Verification items for the finished model (mm, model axes). Face numbers are marked on the shaded views. A direction names the side the tool comes from. Coordinates: 2 decimals unless noted, no trailing zeros. Write each loop counter-clockwise with the first axis right and the second up, starting at its lowest first coordinate (ties: lowest second). Pieces come first, ordered by that corner, then holes. Notation, with made-up numbers: M 57,-36.5 L 91,-36.5 A7 ccw 91,-28.5 Z; hole C 14,-34 d1. An arc over 180 degrees is marked long. One line per item, written item: value.
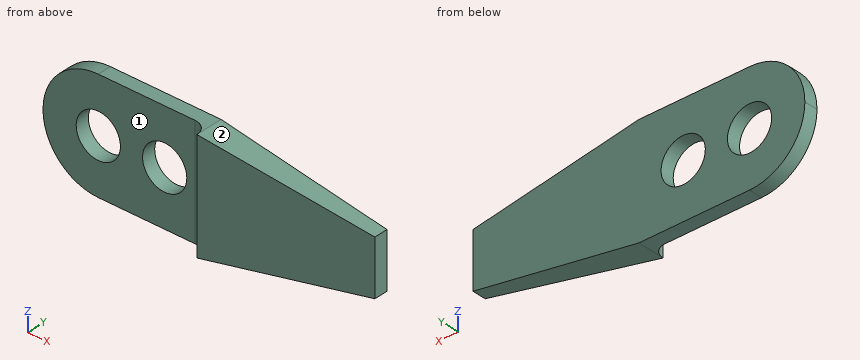
```python
from build123d import *

# Parameters (mm, degrees)
BOSS_EXTRUDE1_DEPTH = 6.35
CUT_EXTRUDE1_DEPTH  = 12.7
FILLET1_R           = 6.35
FILLET2_R           = 1.5875
SKETCH3_R           = 2.54
CUT_EXTRUDE2_DEPTH  = 12.7


with BuildPart() as part:
    # Sketch1 → Boss-Extrude1 (new, symmetric)
    with BuildSketch(Plane.XY):
        Polygon((-19.05, 0), (19.05, 0), (19.05, -1.5875), (0, -3.175), (0, -1.5875), (-19.05, -1.5875), align=None)
    extrude(amount=BOSS_EXTRUDE1_DEPTH, both=True)

    # Sketch2 → Cut-Extrude1 (cut)
    with BuildSketch(Plane(origin=(0, 0, 0), x_dir=(1, 0, 0), z_dir=(0, 1, 0))):
        Polygon((0, 6.35), (19.05, 3.175), (19.05, 6.35), align=None)
    cut_extrude1 = extrude(amount=-CUT_EXTRUDE1_DEPTH, mode=Mode.SUBTRACT)

    # Mirror1: Cut-Extrude1 across plane
    add(cut_extrude1.mirror(Plane.XY), mode=Mode.SUBTRACT)

    # Fillet1
    fillet1_edges = [part.edges().sort_by_distance(p)[0] for p in [
        (-19.05, -0.79375, -6.35),
        (-19.05, -0.79375, 6.35),
    ]]
    fillet(fillet1_edges, radius=FILLET1_R - 0.0001)  # a hair under: the kernel refuses the full size

    # Fillet2
    fillet2_edges = [part.edges().sort_by_distance(p)[0] for p in [
        (0, -1.5875, 0),
    ]]
    fillet(fillet2_edges, radius=FILLET2_R - 0.0001)  # a hair under: the kernel refuses the full size

    # Sketch3 → Cut-Extrude2 (cut)
    with BuildSketch(Plane(origin=(0, 0, 0), x_dir=(1, 0, 0), z_dir=(0, 1, 0))):
        with Locations(Location((-12.7, 0, 0), (0, 0, 270))):
            Circle(SKETCH3_R)
        with Locations(Location((-5.08, 0, 0), (0, 0, 270))):
            Circle(SKETCH3_R)
    extrude(amount=-CUT_EXTRUDE2_DEPTH, mode=Mode.SUBTRACT)


solid = part.part
```
Item 1: Cross-section at B-B, the plane x = -5.08. Enter the section's corners in (y, z), and give its area (3 significant figures).
The answers:
outline: M -1.59,-6.35 L 0,-6.35 L 0,-2.54 L -1.59,-2.54 Z; M -1.59,2.54 L 0,2.54 L 0,6.35 L -1.59,6.35 Z
area: 12.1 mm²
Item 2: Go/stop test with flat-tipped pins: P1, Ø4, axis at x = -12.5, z = -3, coming from the -Y side; P2, Ø4, axis at x = -12.7, z = 0, coming from the -Y side; P3, Ø4, axis at x = 15, z = 3, coming from the -Y side; P4, Ø1.5, axis at y = -1.5, z = 2.5, coming from the -X side. Record where each tip stops, or that it passes through.
The answers:
P1: stops at y = -1.59
P2: passes through
P3: stops at y = -2.09
P4: stops at x = -18.8
Item 3: Cross-section at D-D, the plane x = 14.5. Enter the section's corners in (y, z).
The answers:
outline: M -1.97,-3.93 L 0,-3.93 L 0,3.93 L -1.97,3.93 Z
Item 4: Cross-section at A-A, the plane y = -1.2. Give the number of separate pieces and of enclosed holes in the cut face, and give its area (3 significant figures).
The answers:
separate pieces: 1
enclosed holes: 2
area: 366 mm²
Item 5: Access from +Z, -Z, +X, -X, +Y, -Y to the whole of each face (thin tool, end or side, straight path). Record for the marked faces 1 and 2.
The answers:
face 1: +Z, -Z, -X, -Y
face 2: +Z, +X, +Y, -Y
Item 6: Scan lines: line 1 (X direction, y = -0.35, z = 0); line 2 (X direction, y = -0.25, z = 2); line 3 (Z direction, x = -13, y = -0.25). Record each from-to range of solid material in increasing order.
The answers:
line 1: x = -19.05 to -15.24, -10.16 to -7.62, -2.54 to 19.05
line 2: x = -18.73 to -14.27, -11.13 to -6.65, -3.51 to 19.05
line 3: z = -6.34 to -2.52, 2.52 to 6.34
